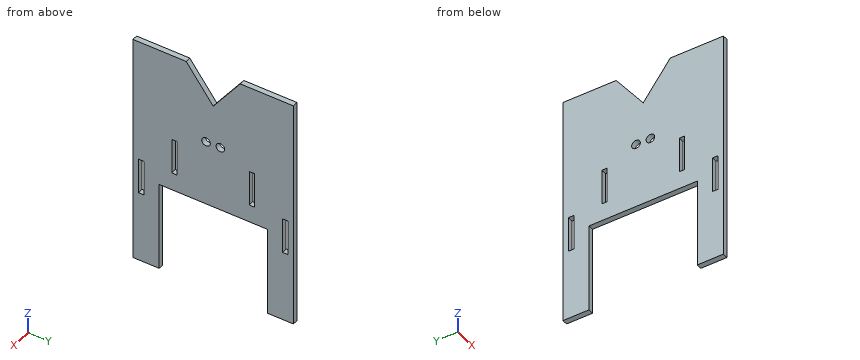
```python
from build123d import *

# Parameters (mm, degrees)
F1_DEPTH = 3
F2_W     = 3
F2_H     = 20
F2_R     = 2.4
F2_W_2   = 60
F2_H_2   = 50
F3_DEPTH = 25


with BuildPart() as f1:
    # F0 (on Right) → F1 (new body)
    with BuildSketch(Plane.YZ):
        Polygon((29.5, 130), (0, 130), (0, 0), (89, 0), (89, 130), (59.5, 130), (44.5, 110), align=None)
    extrude(amount=F1_DEPTH)

    # F2 (on face) → F3 (cut)
    with BuildSketch(Plane.YZ.offset(3)):
        with Locations((4.5, 50)):
            Rectangle(F2_W, F2_H)
        with Locations((84.5, 50)):
            Rectangle(F2_W, F2_H)
        with Locations((40.5, 87)):
            Circle(F2_R)
        with Locations((48.5, 87)):
            Circle(F2_R)
        with Locations((23, 70)):
            Rectangle(F2_W, F2_H)
        with Locations((66, 70)):
            Rectangle(F2_W, F2_H)
        with Locations((44.5, 25)):
            Rectangle(F2_W_2, F2_H_2)
    extrude(amount=-F3_DEPTH, mode=Mode.SUBTRACT)


solid = f1.part
```
Geometry check sheet. Reference: the model listing, model coordinates, mm. Give positions to 0.01 mm unless a question says otherwise; leave off trailing zeros. Write each loop counter-clockwise with the first axis right and the second up, starting at its lowest first coordinate (ties: lowest second). Pieces come first, ordered by that corner, then holes.
1) Section check D-D, the plane y = 48.5. Record the boundary of the cut face in (x, z), and give its area (3 significant figures).
2) Section check B-B, the plane x = 2.25. State how many separate pieces and enclosed holes the cut face has, and give its area (3 significant figures).
3) Section check A-A, the plane z = 87. Record the boundary of the cut face in (x, y), and give its area (3 significant figures).
4) Material ranges on L1, parallel to Y at x = 1.55, z = 59.5; L2, parallel to Y at x = 2.4, z = 30; L3, parallel to Y at x = 2.2, z = 41, recorded low to high.
5) Gauge pin test, flat ends, axial feed: pin 1 (4.5 mm diameter, centred on y = 48.5, z = 87, fed in from +X); pin 2 (0.9 mm diameter, centred on x = 2, y = 39.5, fed in from -Z). Record the tip position at first contact, or that the pin passes through.
6) Section check C-C, the plane z = 11.5. Record the boundary of the cut face in (x, y), and give its area (3 significant figures).
Computed:
1. outline: (0, 50) - (3, 50) - (3, 84.6) - (0, 84.6) - close; (0, 89.4) - (3, 89.4) - (3, 115.33) - (0, 115.33) - close
1. area: 182 mm2
2. separate pieces: 1
2. enclosed holes: 6
2. area: 7,990 mm2
3. outline: (0, 0) - (3, 0) - (3, 38.1) - (0, 38.1) - close; (0, 42.9) - (3, 42.9) - (3, 46.1) - (0, 46.1) - close; (0, 50.9) - (3, 50.9) - (3, 89) - (0, 89) - close
3. area: 238 mm2
4. L1: y = 0 to 3, 6 to 83, 86 to 89
4. L2: y = 0 to 14.5, 74.5 to 89
4. L3: y = 0 to 3, 6 to 14.5, 74.5 to 83, 86 to 89
5. pin 1: passes through
5. pin 2: stops at z = 50
6. outline: (0, 0) - (3, 0) - (3, 14.5) - (0, 14.5) - close; (0, 74.5) - (3, 74.5) - (3, 89) - (0, 89) - close
6. area: 87.0 mm2
